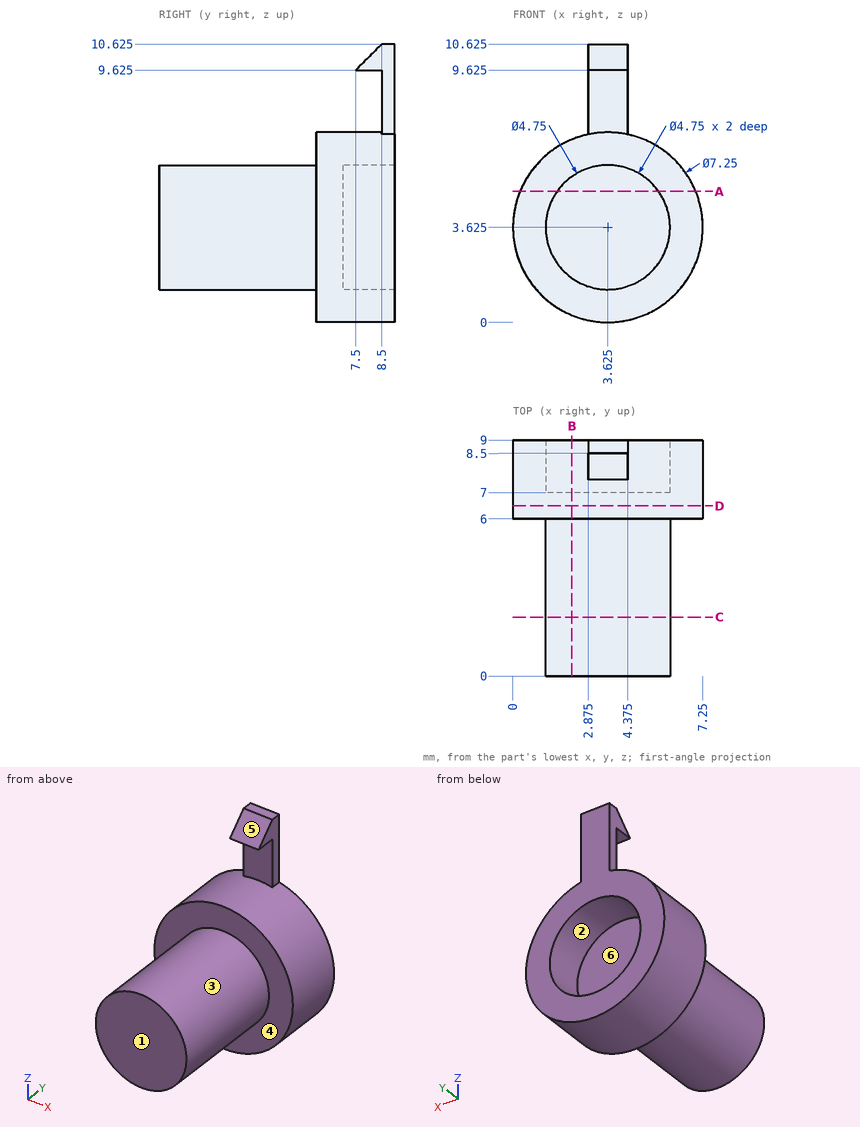
Geometry check sheet. Reference: drawing and pictorial views, mm from the part's lowest x, y, z. A direction names the side the tool comes from. Give positions to 0.01 mm unless a question says otherwise; leave off trailing zeros. Loops run counter-clockwise (first coordinate to the right, second up) from the corner with the lowest first, then second, coordinate; pieces in that order, holes last. Notation, with made-up numbers: (84, 30.25) - (128, 30.25) arc R27 cw to (128, 56.25) - close; hole circle Ø9 at (37, -39.75). An arc over 180 degrees is marked (long way). One line per question, with ' | ' between items. Start each with the question number.
1. Material ranges on line 1 along Y through (x, z) = (3.5, 1.5); line 2 along Y through (x, z) = (6.25, 3); line 3 along X through (y, z) = (8, 1.5), recorded low to high. Write a range as [from, to].
2. Cross-section at B-B, the plane x = 2.25. Enter the section's corners in (y, z), plus the area to 3 significant figures.
3. Set-up check for the marked faces 4, 5 and 6: record each of +Z, -Z, +X, -X, +Y, -Y from which the full face is reachable in a straight line by a thin tool's end or side.
4. Gauge pin test, flat ends, axial feed: pin 1 Ø1.6 at (x, z) = (3.5, 8.5) entering from -Y; pin 2 Ø1.5 at (x, y) = (3, 3.5) entering from -Z; pin 3 Ø1.4 at (x, z) = (4.5, 4.5) entering from +Y. Record the tip position at first contact, or that the pin passes through.
5. Cross-section at D-D, the plane y = 6.5. Enter the section's corners in (x, z) (3 decimals), plus the area to 3 significant figures.
6. Cross-section at C-C, the plane y = 2.25. Enter the section's corners in (x, z) (3 decimals).
7. Cross-section at A-A, the plane z = 5. Enter the section's corners in (x, y), plus the area to 3 significant figures.
8. Draft check along X on the marked faces 1, 2 and 3. Enter one of: released by +X, released by -X, zero draft, split by the parting line, or undercut.
Check result:
1) line 1: y = [0, 7] | line 2: y = [6, 9] | line 3: x = [0.69, 2.56], [4.69, 6.56]
2) outline: (0, 1.69) - (6, 1.69) - (6, 0.27) - (9, 0.27) - (9, 1.69) - (7, 1.69) - (7, 5.56) - (9, 5.56) - (9, 6.98) - (6, 6.98) - (6, 5.56) - (0, 5.56) - close | area: 35.6 mm2
3) face 4: -Y | face 5: +Z, +X, -X, -Y | face 6: +Y
4) pin 1: stops at y = 8.5 | pin 2: stops at z = 1.25 | pin 3: stops at y = 7
5) outline: circle Ø7.25 at (3.625, 3.625) | area: 41.3 mm2
6) outline: circle Ø4.75 at (3.625, 3.625)
7) outline: (0.27, 6) - (1.69, 6) - (1.69, 0) - (5.56, 0) - (5.56, 6) - (6.98, 6) - (6.98, 9) - (5.56, 9) - (5.56, 7) - (1.69, 7) - (1.69, 9) - (0.27, 9) - close | area: 35.6 mm2
8) face 1: zero draft | face 2: undercut | face 3: split by the parting line
